Could you check a few things on this drawing? It's one solid part, dimensions in mm from its lowest x, y, z. A direction names the side the tool comes from. Give positions to 0.01 mm unless a question says otherwise; leave off trailing zeros. Write each loop counter-clockwise with the first axis right and the second up, starting at its lowest first coordinate (ties: lowest second). Pieces come first, ordered by that corner, then holes. Notation, with made-up numbers: M -39,80.25 L 14,80.25 A19 ccw 14,104.25 Z; hole C 40.25,19.25 d8. An arc over 180 degrees is marked long. Answer as CSV lines item,"result". Start each with the question number.
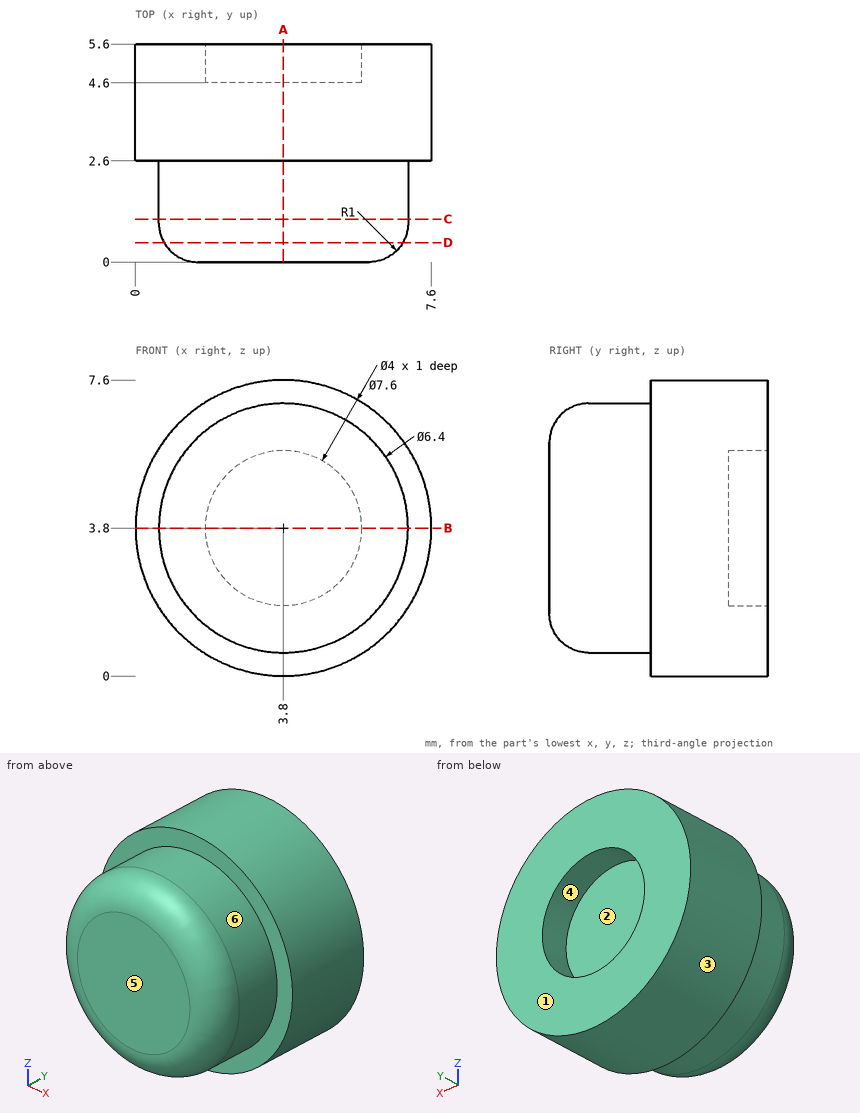
1) Thinking about a two-plate mould opening in Z: for the marked faces 1, 2, 3 and 4, which applies, released by +Z, released by -Z, zero draft, split by the parting line, or undercut?
2) On a 3-axis mill with a long thin cutter (end or side, diameter ignored), from which of +Z, -Z, +X, -X, +Y, -Y can I reach the whole of each face in a straight line? I mean the marked faces 5 and 6. Say none if no direction works.
3) I'm going to push flat-ended pins straight in: P1, Ø1, axis at x = 1.5, y = 5, coming from the -Z side; P2, Ø1, axis at y = 1.5, z = 3, coming from the -X side. Where does each tip first touch, or does it pass through?
4) I want a section at D-D, the plane y = 0.5. Please give me the cut outline in (x, z), then the cut area to 3 significant figures.
5) I want a section at B-B, the plane z = 3.8. Please give me the cut outline in (x, y).
6) I want a section at A-A, the plane x = 3.8. Please give me the cut outline in (y, z), then the cut area to 3 significant figures.
7) I need wall thicknesses on L1, parallel to Z at x = 3.8, y = 5.2; L2, parallel to Y at x = 3.5, z = 0.5. Which ranges of each line are inside material? Lowest first, please. Write a range as from..to.
8) I want a section at C-C, the plane y = 1.1. Please give me the cut outline in (x, z).
Values found:
1,face 1,"zero draft"
1,face 2,"undercut"
1,face 3,"split by the parting line"
1,face 4,"undercut"
2,face 5,"+Z, -Z, +X, -X, -Y"
2,face 6,"-Y"
3,P1,"stops at z = 0.45"
3,P2,"stops at x = 0.61"
4,outline,"C 3.8,3.8 d6.13"
4,area,"29.5 mm²"
5,outline,"M 0,2.6 L 0.6,2.6 L 0.6,1 A1 ccw 1.6,0 L 6,0 A1 ccw 7,1 L 7,2.6 L 7.6,2.6 L 7.6,5.6 L 5.8,5.6 L 5.8,4.6 L 1.8,4.6 L 1.8,5.6 L 0,5.6 Z"
6,outline,"M 0,1.6 A1 ccw 1,0.6 L 2.6,0.6 L 2.6,0 L 5.6,0 L 5.6,1.8 L 4.6,1.8 L 4.6,5.8 L 5.6,5.8 L 5.6,7.6 L 2.6,7.6 L 2.6,7 L 1,7 A1 ccw 0,6 Z"
6,area,"35.0 mm²"
7,L1,"z = 0..1.8, 5.8..7.6"
7,L2,"y = 2.6..5.6"
8,outline,"C 3.8,3.8 d6.4"
